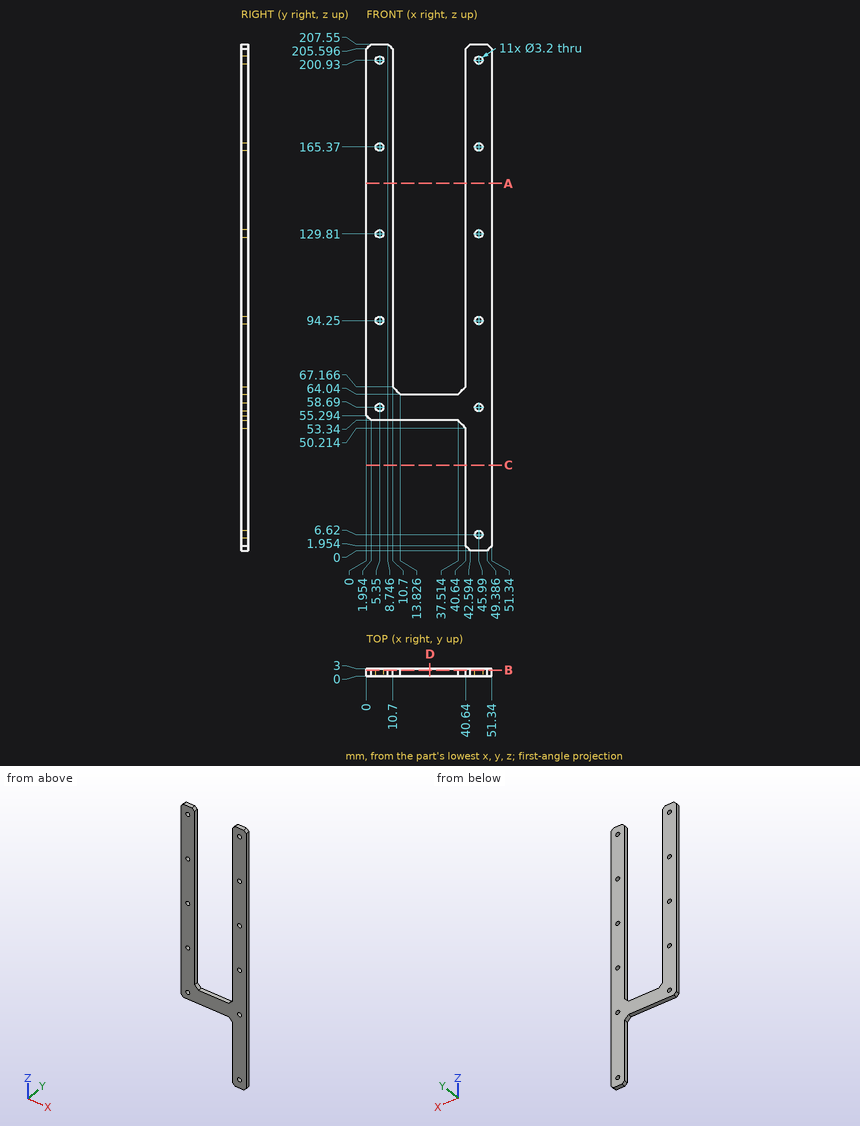
Study the drawing (mm; zero at the part's minimum x, y, z) and answer. Coordinates: 2 decimals unless noted, no trailing zeros. Loops run counter-clockwise (first coordinate to the right, second up) from the corner with the lowest first, then second, coordinate; pieces in that order, holes last. Notation, with made-up numbers: (-36.5, 83) -> (-9.5, 83) arc R19 ccw to (-9.5, 99) -> close; hole circle Ø7 at (44, -34). An arc over 180 degrees is marked (long way). Answer in a Markdown table with one row per item. Add a question column.
1. The part is cut by section D-D, the plane x = 26. Write down the section's boundary in (y, z), then the cut area to 3 significant figures.
2. The part is cut by section C-C, the plane z = 35. Write down the section's boundary in (x, y), then the cut area to 3 significant figures.
3. Consider line 1 (X direction, y = 0.95, z = 200.93); line 2 (X direction, y = 2.45, z = 196); line 3 (Z direction, x = 3, y = 1.15). Determine where each line is inside the solid, lowest interval first. Write a range as [from, to].
4. The part is cut by section B-B, the plane y = 2.45. Count the separate pieces of the cut face and the enclosed holes in it, then the cut area to 3 significant figures.
5. Flat-ended cylindrical pins translate along their axes: P1, Ø1, axis at x = 32.5, y = 1, coming from the -Z side; P2, Ø0.9, axis at y = 1, z = 17, coming from the -X side; P3, Ø1.5, axis at x = 23, y = 1.5, coming from the +Z side. Find the tip coordinate at first contact, or state that the pin passes through.
6. The part is cut by section A-A, the plane z = 150.5. Write down the section's boundary in (x, y).
Answer below:
| question | item | result |
|---|---|---|
| 1 | outline | (0, 53.34) -> (3, 53.34) -> (3, 64.04) -> (0, 64.04) -> close |
| 1 | area | 32.1 mm2 |
| 2 | outline | (40.64, 0) -> (51.34, 0) -> (51.34, 3) -> (40.64, 3) -> close |
| 2 | area | 32.1 mm2 |
| 3 | line 1 | [0, 3.75], [6.95, 10.7], [40.64, 44.39], [47.59, 51.34] |
| 3 | line 2 | [0, 10.7], [40.64, 51.34] |
| 3 | line 3 | [53.34, 207.55] |
| 4 | separate pieces | 1 |
| 4 | enclosed holes | 11 |
| 4 | area | 4,100 mm2 |
| 5 | P1 | z = 53.34 |
| 5 | P2 | x = 40.64 |
| 5 | P3 | z = 64.04 |
| 6 | outline | (0, 0) -> (10.7, 0) -> (10.7, 3) -> (0, 3) -> close; (40.64, 0) -> (51.34, 0) -> (51.34, 3) -> (40.64, 3) -> close |
